from build123d import *

# Parameters (mm, degrees)
SALIENTE_EXTRUIR1_DEPTH = 72
CROQUIS2_R              = 1.5
CORTAR_EXTRUIR1_DEPTH   = 73
CROQUIS3_R              = 1.5
CORTAR_EXTRUIR2_DEPTH   = 11


with BuildPart() as part:
    # Croquis1 → Saliente-Extruir1 (new body)
    with BuildSketch(Plane.XY):
        with BuildLine():
            Line((0, 0), (10, 0))
            Line((10, 0), (10, 75))
            Line((10, 75), (0, 75))
            Line((0, 75), (0, 45.65))
            ThreePointArc((0, 45.65), (8.15, 37.5), (0, 29.35))
            Line((0, 29.35), (0, 0))
        make_face()
    extrude(amount=SALIENTE_EXTRUIR1_DEPTH)

    # Croquis2 → Cortar-Extruir1 (cut, through all)
    with BuildSketch(Plane.XY.offset(72)):
        with Locations((4, 63)):
            Circle(CROQUIS2_R)
        with Locations((4, 12)):
            Circle(CROQUIS2_R)
    extrude(amount=-CORTAR_EXTRUIR1_DEPTH, mode=Mode.SUBTRACT)

    # Croquis3 → Cortar-Extruir2 (cut, through all)
    with BuildSketch(Plane(origin=(10, 0, 0), x_dir=(0, 0, -1), z_dir=(1, 0, 0))):
        with Locations(Location((-36, 37.5, 0), (0, 0, 90))):  # turned: the seam where the file's is
            Circle(CROQUIS3_R)
    extrude(amount=-CORTAR_EXTRUIR2_DEPTH, mode=Mode.SUBTRACT)


solid = part.part
CAD build for the part. Positions are in the model's coordinates, mm. Round coordinates to 2 decimals unless told otherwise and drop trailing zeros. Loops run counter-clockwise (first coordinate to the right, second up) from the corner with the lowest first, then second, coordinate; pieces in that order, holes last. Notation, with made-up numbers: (-22, -23.75) - (37, -23.75) arc R17 cw to (37, -11.75) - close; hole circle Ø4 at (83, 29.5). An arc over 180 degrees is marked (long way). Put each result on its own line as item: value.
1. Slice it at B-B on y = 37.5. List the corners of the cut face in (x, z).
Geometry check:
outline: (8.15, 0) - (10, 0) - (10, 34.5) - (8.15, 34.5) - close; (8.15, 37.5) - (10, 37.5) - (10, 72) - (8.15, 72) - close
2. Slice it at C-C on x = 4. List the corners of the cut face in (y, z).
Geometry check:
outline: (0, 0) - (10.5, 0) - (10.5, 72) - (0, 72) - close; (13.5, 0) - (30.4, 0) - (30.4, 72) - (13.5, 72) - close; (44.6, 0) - (61.5, 0) - (61.5, 72) - (44.6, 72) - close; (64.5, 0) - (75, 0) - (75, 72) - (64.5, 72) - close
3. Slice it at D-D on y = 63. List the corners of the cut face in (x, z), and give its area (3 significant figures).
Geometry check:
outline: (0, 0) - (2.5, 0) - (2.5, 72) - (0, 72) - close; (5.5, 0) - (10, 0) - (10, 72) - (5.5, 72) - close
area: 504 mm²
4. Two-plate mould, pull along Y, no slides. Class faces 1 (the cylindrical face through (5.386, 11.425, 36.504)), 2 (the flat face through (5, 0, 35)), 3 (the flat face through (10, 37, 43)): released by +Y, released by -Y, zero draft, split by the parting line, or undercut.
Geometry check:
face 1: undercut
face 2: released by -Y
face 3: zero draft
5. Slice it at A-A on z = 11. List the corners of the cut face in (x, y).
Geometry check:
outline: (0, 0) - (10, 0) - (10, 75) - (0, 75) - (0, 45.65) arc R8.15 cw to (0, 29.35) - close; hole circle Ø3 at (4, 12); hole circle Ø3 at (4, 63)
6. Pin check, flat tips, straight feed: P1, Ø5, axis at y = 37.5, z = 36, coming from the -X side; P2, Ø1, axis at y = 38.5, z = 17, coming from the -X side. Stop position of each tip, or through.
Geometry check:
P1: x = 7.76
P2: x = 8.01
7. Wall check: line 1 (Z direction, x = 9.65, y = 37.5); line 2 (Y direction, x = 8.75, z = 36); line 3 (Y direction, x = 3.25, z = 5). Give the ranges that are in metal, low to high.
Geometry check:
line 1: 0 to 34.5, 37.5 to 72
line 2: 0 to 36, 39 to 75
line 3: 0 to 10.7, 13.3 to 30.03, 44.97 to 61.7, 64.3 to 75
